from build123d import *

# Parameters (mm, degrees)
SKETCH_1_R      = 10
EXTRUDE_1_DEPTH = 10
SKETCH_2_R      = 6.599829968
EXTRUDE_2_DEPTH = 20


with BuildPart() as part:
    # 草图1 → 凸台-拉伸1 (new body)
    with BuildSketch(Plane.XY):
        with BuildLine():
            Line((24.803918541, -3.125), (19.843134833, -42.5))
            ThreePointArc((19.843134833, -42.5), (-2.812850316, -59.80120888), (-19.754350787, -36.875))
            ThreePointArc((-19.754350787, -36.875), (-19.502870979, -23.051442481), (-23.046742584, -9.6875))
            ThreePointArc((-23.046742584, -9.6875), (-3.396839472, 24.768154586), (24.803918541, -3.125))
        make_face()
        Circle(SKETCH_1_R, mode=Mode.SUBTRACT)
    extrude(amount=EXTRUDE_1_DEPTH)

    # 草图2 → 凸台-拉伸2 (add)
    with BuildSketch(Plane(origin=(0, 0, 0), x_dir=(-1, 0, 0), z_dir=(0, 0, -1))):
        with Locations((0, -43.431952643)):
            Circle(SKETCH_2_R)
    extrude(amount=EXTRUDE_2_DEPTH)


solid = part.part
CAD build for the part. Positions are in the model's coordinates, mm. A direction names the side the tool comes from. Give positions to 0.01 mm unless a question says otherwise; leave off trailing zeros. Loops run counter-clockwise (first coordinate to the right, second up) from the corner with the lowest first, then second, coordinate; pieces in that order, holes last. Notation, with made-up numbers: M 15,80.5 L 57,80.5 A25 cw 57,119.5 Z; hole C -27,45 d7. An arc over 180 degrees is marked long. Answer in a Markdown table with one row per item. Add a question column.
Item 1: Band-saw the part on D-D on y = -48. Give the cut face in (x, z), then the cut area to 3 significant figures.
Item 2: Mould opens along X. For faces 1 (the face through (-4.031, 24.673, 4.93)), 2 (the face through (22.358, -22.537, 4.93)), 3 (the face through (-2.17, -9.76, 4.93)) say: +X half, -X half, draft (parallel to the pull), parting line (faces both ways), or undercut.
Item 3: Drop flat-ended pins along their axis: P1, Ø8, axis at x = 7.5, z = 6, coming from the +Y side; P2, Ø10, axis at x = 17.5, z = 0.5, coming from the -Y side; P3, Ø4, axis at y = 6.5, z = 7, coming from the +X side; P4, Ø16, axis at x = 0, y = 0, coming from the +Z side. Give the stop position or say it passes through.
Item 4: Band-saw the part on C-C on z = 4.5. Give the cut face in (x, y) (1 decimal), then the cut area to 3 significant figures.
Item 5: Probe probe 1 along Y at (x, z) = (0, 3); probe 2 along Z at (x, y) = (-9.5, 6.5); probe 3 along Y at (x, z) = (4, 4.75). List the from-to ranges inside material, lowest first.
Item 6: Band-saw the part on A-A on y = 0. Give the cut face in (x, z).
Item 7: Tool access for faces 4 (the face through (-19.48, -23.24, 4.93)), 5 (the face through (-3.55, -37.87, -9.86)): list every direction of +Z, -Z, +X, -X, +Y, -Y with a clear straight run to the whole face (end or side of a thin tool).
Item 8: Band-saw the part on B-B on x = 0. Give the cut face in (y, z).
Reply:
| question | item | result |
|---|---|---|
| 1 | outline | M -18.33,0 L -4.76,0 L -4.76,-20 L 4.76,-20 L 4.76,0 L 18.33,0 L 18.33,10 L -18.33,10 Z |
| 1 | area | 557 mm^2 |
| 2 | face 1 | parting line |
| 2 | face 2 | +X half |
| 2 | face 3 | undercut |
| 3 | P1 | stops at y = 24.75 |
| 3 | P2 | stops at y = -55.61 |
| 3 | P3 | stops at x = 24.59 |
| 3 | P4 | passes through |
| 4 | outline | M -23,-9.7 A50 cw -19.8,-36.9 A20 ccw long 19.8,-42.5 L 24.8,-3.1 A25 ccw long Z; hole C 0,0 d20 |
| 4 | area | 3,050 mm^2 |
| 5 | probe 1 | y = -60 to -10, 10 to 25 |
| 5 | probe 2 | z = 0 to 10 |
| 5 | probe 3 | y = -59.6 to -9.17, 9.17 to 24.68 |
| 6 | outline | M -25,0 L -10,0 L -10,10 L -25,10 Z; M 10,0 L 25,0 L 25,10 L 10,10 Z |
| 7 | face 4 | +Z, -Z, -X |
| 7 | face 5 | -Z |
| 8 | outline | M -60,0 L -50.03,0 L -50.03,-20 L -36.83,-20 L -36.83,0 L -10,0 L -10,10 L -60,10 Z; M 10,0 L 25,0 L 25,10 L 10,10 Z |
